```python
from build123d import *

# Parameters (mm, degrees)
SKETCH1_W           = 150
SKETCH1_H           = 160
BOSS_EXTRUDE1_DEPTH = 3.2
CUT_EXTRUDE1_REACH  = 5.2
SKETCH2_R           = 25
CUT_EXTRUDE2_REACH  = 5.2
SKETCH3_R           = 2.75


with BuildPart() as part:
    # Sketch1 → Boss-Extrude1 (new body)
    with BuildSketch(Plane.XY):
        Rectangle(SKETCH1_W, SKETCH1_H)
    extrude(amount=BOSS_EXTRUDE1_DEPTH)

    # Sketch2 → Cut-Extrude1 (cut, up to next)
    with BuildSketch(Plane.XY.offset(3.2), mode=Mode.PRIVATE) as cut_extrude1_sk1:
        with Locations((0, -12)):
            Circle(SKETCH2_R)
    cut_extrude1_tool1 = extrude(cut_extrude1_sk1.sketch, amount=-CUT_EXTRUDE1_REACH, mode=Mode.PRIVATE) & part.part
    add(cut_extrude1_tool1.solids().sort_by_distance((0, -12, 3.2))[0], mode=Mode.SUBTRACT)

    # Sketch3 → Cut-Extrude2 (cut, up to next)
    with BuildSketch(Plane(origin=(0, 0, 0), x_dir=(-1, 0, 0), z_dir=(0, 0, -1)), mode=Mode.PRIVATE) as cut_extrude2_sk1:
        with Locations((65, 24)):
            Circle(SKETCH3_R)
    cut_extrude2_tool1 = extrude(cut_extrude2_sk1.sketch, amount=-CUT_EXTRUDE2_REACH, mode=Mode.PRIVATE) & part.part
    add(cut_extrude2_tool1.solids().sort_by_distance((-65, 24, 0))[0], mode=Mode.SUBTRACT)
    # Sketch3 → Cut-Extrude2 (cut, up to next)
    with BuildSketch(Plane(origin=(0, 0, 0), x_dir=(-1, 0, 0), z_dir=(0, 0, -1)), mode=Mode.PRIVATE) as cut_extrude2_sk2:
        with Locations((-70, -75)):
            Circle(SKETCH3_R)
    cut_extrude2_tool2 = extrude(cut_extrude2_sk2.sketch, amount=-CUT_EXTRUDE2_REACH, mode=Mode.PRIVATE) & part.part
    add(cut_extrude2_tool2.solids().sort_by_distance((70, -75, 0))[0], mode=Mode.SUBTRACT)
    # Sketch3 → Cut-Extrude2 (cut, up to next)
    with BuildSketch(Plane(origin=(0, 0, 0), x_dir=(-1, 0, 0), z_dir=(0, 0, -1)), mode=Mode.PRIVATE) as cut_extrude2_sk3:
        with Locations((36, -75)):
            Circle(SKETCH3_R)
    cut_extrude2_tool3 = extrude(cut_extrude2_sk3.sketch, amount=-CUT_EXTRUDE2_REACH, mode=Mode.PRIVATE) & part.part
    add(cut_extrude2_tool3.solids().sort_by_distance((-36, -75, 0))[0], mode=Mode.SUBTRACT)
    # Sketch3 → Cut-Extrude2 (cut, up to next)
    with BuildSketch(Plane(origin=(0, 0, 0), x_dir=(-1, 0, 0), z_dir=(0, 0, -1)), mode=Mode.PRIVATE) as cut_extrude2_sk4:
        with Locations((-36, -75)):
            Circle(SKETCH3_R)
    cut_extrude2_tool4 = extrude(cut_extrude2_sk4.sketch, amount=-CUT_EXTRUDE2_REACH, mode=Mode.PRIVATE) & part.part
    add(cut_extrude2_tool4.solids().sort_by_distance((36, -75, 0))[0], mode=Mode.SUBTRACT)
    # Sketch3 → Cut-Extrude2 (cut, up to next)
    with BuildSketch(Plane(origin=(0, 0, 0), x_dir=(-1, 0, 0), z_dir=(0, 0, -1)), mode=Mode.PRIVATE) as cut_extrude2_sk5:
        with Locations((70, -75)):
            Circle(SKETCH3_R)
    cut_extrude2_tool5 = extrude(cut_extrude2_sk5.sketch, amount=-CUT_EXTRUDE2_REACH, mode=Mode.PRIVATE) & part.part
    add(cut_extrude2_tool5.solids().sort_by_distance((-70, -75, 0))[0], mode=Mode.SUBTRACT)
    # Sketch3 → Cut-Extrude2 (cut, up to next)
    with BuildSketch(Plane(origin=(0, 0, 0), x_dir=(-1, 0, 0), z_dir=(0, 0, -1)), mode=Mode.PRIVATE) as cut_extrude2_sk6:
        with Locations((-70, -40)):
            Circle(SKETCH3_R)
    cut_extrude2_tool6 = extrude(cut_extrude2_sk6.sketch, amount=-CUT_EXTRUDE2_REACH, mode=Mode.PRIVATE) & part.part
    add(cut_extrude2_tool6.solids().sort_by_distance((70, -40, 0))[0], mode=Mode.SUBTRACT)
    # Sketch3 → Cut-Extrude2 (cut, up to next)
    with BuildSketch(Plane(origin=(0, 0, 0), x_dir=(-1, 0, 0), z_dir=(0, 0, -1)), mode=Mode.PRIVATE) as cut_extrude2_sk7:
        with Locations((-70, 25)):
            Circle(SKETCH3_R)
    cut_extrude2_tool7 = extrude(cut_extrude2_sk7.sketch, amount=-CUT_EXTRUDE2_REACH, mode=Mode.PRIVATE) & part.part
    add(cut_extrude2_tool7.solids().sort_by_distance((70, 25, 0))[0], mode=Mode.SUBTRACT)
    # Sketch3 → Cut-Extrude2 (cut, up to next)
    with BuildSketch(Plane(origin=(0, 0, 0), x_dir=(-1, 0, 0), z_dir=(0, 0, -1)), mode=Mode.PRIVATE) as cut_extrude2_sk8:
        with Locations((-36, 75)):
            Circle(SKETCH3_R)
    cut_extrude2_tool8 = extrude(cut_extrude2_sk8.sketch, amount=-CUT_EXTRUDE2_REACH, mode=Mode.PRIVATE) & part.part
    add(cut_extrude2_tool8.solids().sort_by_distance((36, 75, 0))[0], mode=Mode.SUBTRACT)
    # Sketch3 → Cut-Extrude2 (cut, up to next)
    with BuildSketch(Plane(origin=(0, 0, 0), x_dir=(-1, 0, 0), z_dir=(0, 0, -1)), mode=Mode.PRIVATE) as cut_extrude2_sk9:
        with Locations((36, 75)):
            Circle(SKETCH3_R)
    cut_extrude2_tool9 = extrude(cut_extrude2_sk9.sketch, amount=-CUT_EXTRUDE2_REACH, mode=Mode.PRIVATE) & part.part
    add(cut_extrude2_tool9.solids().sort_by_distance((-36, 75, 0))[0], mode=Mode.SUBTRACT)
    # Sketch3 → Cut-Extrude2 (cut, up to next)
    with BuildSketch(Plane(origin=(0, 0, 0), x_dir=(-1, 0, 0), z_dir=(0, 0, -1)), mode=Mode.PRIVATE) as cut_extrude2_sk10:
        with Locations((65, 75)):
            Circle(SKETCH3_R)
    cut_extrude2_tool10 = extrude(cut_extrude2_sk10.sketch, amount=-CUT_EXTRUDE2_REACH, mode=Mode.PRIVATE) & part.part
    add(cut_extrude2_tool10.solids().sort_by_distance((-65, 75, 0))[0], mode=Mode.SUBTRACT)
    # Sketch3 → Cut-Extrude2 (cut, up to next)
    with BuildSketch(Plane(origin=(0, 0, 0), x_dir=(-1, 0, 0), z_dir=(0, 0, -1)), mode=Mode.PRIVATE) as cut_extrude2_sk11:
        with Locations((70, -40)):
            Circle(SKETCH3_R)
    cut_extrude2_tool11 = extrude(cut_extrude2_sk11.sketch, amount=-CUT_EXTRUDE2_REACH, mode=Mode.PRIVATE) & part.part
    add(cut_extrude2_tool11.solids().sort_by_distance((-70, -40, 0))[0], mode=Mode.SUBTRACT)
    # Sketch3 → Cut-Extrude2 (cut, up to next)
    with BuildSketch(Plane(origin=(0, 0, 0), x_dir=(-1, 0, 0), z_dir=(0, 0, -1)), mode=Mode.PRIVATE) as cut_extrude2_sk12:
        with Locations((70, -6)):
            Circle(SKETCH3_R)
    cut_extrude2_tool12 = extrude(cut_extrude2_sk12.sketch, amount=-CUT_EXTRUDE2_REACH, mode=Mode.PRIVATE) & part.part
    add(cut_extrude2_tool12.solids().sort_by_distance((-70, -6, 0))[0], mode=Mode.SUBTRACT)
    # Sketch3 → Cut-Extrude2 (cut, up to next)
    with BuildSketch(Plane(origin=(0, 0, 0), x_dir=(-1, 0, 0), z_dir=(0, 0, -1)), mode=Mode.PRIVATE) as cut_extrude2_sk13:
        with Locations((0, 75)):
            Circle(SKETCH3_R)
    cut_extrude2_tool13 = extrude(cut_extrude2_sk13.sketch, amount=-CUT_EXTRUDE2_REACH, mode=Mode.PRIVATE) & part.part
    add(cut_extrude2_tool13.solids().sort_by_distance((0, 75, 0))[0], mode=Mode.SUBTRACT)
    # Sketch3 → Cut-Extrude2 (cut, up to next)
    with BuildSketch(Plane(origin=(0, 0, 0), x_dir=(-1, 0, 0), z_dir=(0, 0, -1)), mode=Mode.PRIVATE) as cut_extrude2_sk14:
        with Locations((-61.592770869, 55.875856237)):
            Circle(SKETCH3_R)
    cut_extrude2_tool14 = extrude(cut_extrude2_sk14.sketch, amount=-CUT_EXTRUDE2_REACH, mode=Mode.PRIVATE) & part.part
    add(cut_extrude2_tool14.solids().sort_by_distance((61.592771, 55.875856, 0))[0], mode=Mode.SUBTRACT)


solid = part.part
```
Input: part model. Units: mm. Frame: model coordinates. Round coordinates to 2 decimals unless told otherwise and drop trailing zeros. Loops run counter-clockwise (first coordinate to the right, second up) from the corner with the lowest first, then second, coordinate; pieces in that order, holes last. Notation, with made-up numbers: (65, -1) -> (101, -1) arc R22 cw to (101, 29) -> close; hole circle Ø7 at (38, 8). An arc over 180 degrees is marked (long way). Write each question's results on one line, items separated by ' | '.
1. Section C-C (y = 75). Return loops of the section in (x, z).
Geometry results:
outline: (-75, 0) -> (-67.75, 0) -> (-67.75, 3.2) -> (-75, 3.2) -> close; (-62.25, 0) -> (-38.75, 0) -> (-38.75, 3.2) -> (-62.25, 3.2) -> close; (-33.25, 0) -> (-2.75, 0) -> (-2.75, 3.2) -> (-33.25, 3.2) -> close; (2.75, 0) -> (33.25, 0) -> (33.25, 3.2) -> (2.75, 3.2) -> close; (38.75, 0) -> (75, 0) -> (75, 3.2) -> (38.75, 3.2) -> close
2. Section B-B (y = -12). Return loops of the section in (x, z), and give its area (3 significant figures).
Geometry results:
outline: (-75, 0) -> (-25, 0) -> (-25, 3.2) -> (-75, 3.2) -> close; (25, 0) -> (75, 0) -> (75, 3.2) -> (25, 3.2) -> close | area: 320 mm2
3. Section A-A (x = 0). Return loops of the section in (y, z), and give its area (3 significant figures).
Geometry results:
outline: (-80, 0) -> (-37, 0) -> (-37, 3.2) -> (-80, 3.2) -> close; (13, 0) -> (72.25, 0) -> (72.25, 3.2) -> (13, 3.2) -> close; (77.75, 0) -> (80, 0) -> (80, 3.2) -> (77.75, 3.2) -> close | area: 334 mm2
4. First-contact query: P1, Ø5, axis at x = -70, y = -40, coming from the +Z side. Flat tip, straight axial feed; report the tip coordinate or a pass-through.
Geometry results:
P1: through
5. Ray query, line 1 (Y direction, x = -70, z = 0.85); line 2 (Y direction, x = -36, z = 2.05); line 3 (Y direction, x = 70, z = 1.6). Return the intervals inside material, ascending. Write a range as from..to.
Geometry results:
line 1: -80..-77.75, -72.25..-42.75, -37.25..-8.75, -3.25..80 | line 2: -80..-77.75, -72.25..72.25, 77.75..80 | line 3: -80..-77.75, -72.25..-42.75, -37.25..22.25, 27.75..80
6. Mould query, pull axis Y, two halves, no side actions, for faces 1 (the face through (23.846, -4.491, 1.622)), 2 (the face through (-1, 19, 0)). Classes: +Y half, -Y half, draft (parallel to the pull), parting line (faces both ways), or undercut.
Geometry results:
face 1: undercut | face 2: draft
7. Section D-D (z = 0.95). State how many separate pieces and enclosed holes the cut face has, and give its area (3 significant figures).
Geometry results:
separate pieces: 1 | enclosed holes: 15 | area: 21,700 mm2
